```python
from build123d import *

# Parameters (mm, degrees)
SKETCH_1_W                    = 28.5
SKETCH_1_H                    = 8.75
EXTRUDE_1_DEPTH               = 1
HOLE_WIZARD_M10_1_D           = 11
HOLE_WIZARD_M10_1_CBORE_D     = 28.5
HOLE_WIZARD_M10_1_CBORE_DEPTH = 6.75
HOLE_WIZARD_2_5_2_5_1_D       = 2.5
HOLE_WIZARD_2_5_2_5_1_DEPTH   = 19.25
FILLET_1_R                    = 1


with BuildPart() as part:
    # 草图1 → 旋转1 (revolve)
    with BuildSketch(Plane.XZ, mode=Mode.PRIVATE) as revolve_1_sk:
        with Locations((14.25, 4.375)):
            Rectangle(SKETCH_1_W, SKETCH_1_H)
    revolve(revolve_1_sk.sketch.rotate(Axis((0, 0, 8.75), (0, 0, -1)), 180), axis=Axis((0, 0, 8.75), (0, 0, -1)))

    # 草图2 → 凸台-拉伸1 (add)
    with BuildSketch(Plane.XY.offset(8.75)):
        with BuildLine():
            Line((-8.705372964, 19.931858457), (-8.056820792, 17.511428803))
            ThreePointArc((-8.056820792, 17.511428803), (-5.758723754, 21.491849635), (-1.778302922, 19.193752596))
            Line((-1.778302922, 19.193752596), (-2.426855093, 21.614182251))
            ThreePointArc((-2.426855093, 21.614182251), (10.875, 18.836052532), (19.931858457, 8.705372964))
            Line((19.931858457, 8.705372964), (17.511428803, 8.056820792))
            ThreePointArc((17.511428803, 8.056820792), (21.491849635, 5.758723754), (19.193752596, 1.778302922))
            Line((19.193752596, 1.778302922), (21.614182251, 2.426855093))
            ThreePointArc((21.614182251, 2.426855093), (18.836052532, -10.875), (8.705372964, -19.931858457))
            Line((8.705372964, -19.931858457), (8.056820792, -17.511428803))
            ThreePointArc((8.056820792, -17.511428803), (5.758723754, -21.491849635), (1.778302922, -19.193752596))
            Line((1.778302922, -19.193752596), (2.426855093, -21.614182251))
            ThreePointArc((2.426855093, -21.614182251), (-10.875, -18.836052532), (-19.931858457, -8.705372964))
            Line((-19.931858457, -8.705372964), (-17.511428803, -8.056820792))
            ThreePointArc((-17.511428803, -8.056820792), (-21.491849635, -5.758723754), (-19.193752596, -1.778302922))
            Line((-19.193752596, -1.778302922), (-21.614182251, -2.426855093))
            ThreePointArc((-21.614182251, -2.426855093), (-18.836052532, 10.875), (-8.705372964, 19.931858457))
        make_face()
    extrude(amount=EXTRUDE_1_DEPTH)

    # 草图3 → 旋转2 (revolve)
    with BuildSketch(Plane.XZ, mode=Mode.PRIVATE) as revolve_2_sk:
        Polygon((8.5, 19.25), (0, 19.25), (0, 9.75), (9.5, 9.75), (9.5, 14.25), (8.5, 14.25), align=None)
    revolve(revolve_2_sk.sketch.rotate(Axis((0, 0, 19.25), (0, 0, -1)), 180), axis=Axis((0, 0, 19.25), (0, 0, -1)))

    # 草图4 → 切除-旋转1 (revolve, cut)
    with BuildSketch(Plane(origin=(0, -18.352590699, 0), x_dir=(1, 0, 0), z_dir=(0, 1, 0))):
        Polygon((6.617561857, 0), (4.917561857, 0), (4.917561857, -9.75), (8.167561857, -9.75), (8.167561857, -2.5), (6.617561857, -2.5), align=None)
    revolve(axis=Axis((4.917561857, -18.352590699, 0), (0, 0, 1)), mode=Mode.SUBTRACT)

    # 草图5 → 切除-旋转2 (revolve, cut)
    with BuildSketch(Plane(origin=(0, -4.917561857, 0), x_dir=(1, 0, 0), z_dir=(0, 1, 0))):
        Polygon((-16.652590699, 0), (-18.352590699, 0), (-18.352590699, -9.75), (-15.102590699, -9.75), (-15.102590699, -2.5), (-16.652590699, -2.5), align=None)
    revolve(axis=Axis((-18.352590699, -4.917561857, 0), (0, 0, 1)), mode=Mode.SUBTRACT)

    # 草图6 → 切除-旋转3 (revolve, cut)
    with BuildSketch(Plane(origin=(0, 18.352590699, 0), x_dir=(1, 0, 0), z_dir=(0, 1, 0))):
        Polygon((-3.217561857, 0), (-4.917561857, 0), (-4.917561857, -9.75), (-1.667561857, -9.75), (-1.667561857, -2.5), (-3.217561857, -2.5), align=None)
    revolve(axis=Axis((-4.917561857, 18.352590699, 0), (0, 0, 1)), mode=Mode.SUBTRACT)

    # 草图7 → 切除-旋转4 (revolve, cut)
    with BuildSketch(Plane(origin=(0, 4.917561857, 0), x_dir=(1, 0, 0), z_dir=(0, 1, 0))):
        Polygon((20.052590699, 0), (18.352590699, 0), (18.352590699, -9.75), (21.602590699, -9.75), (21.602590699, -2.5), (20.052590699, -2.5), align=None)
    revolve(axis=Axis((18.352590699, 4.917561857, 0), (0, 0, 1)), mode=Mode.SUBTRACT)

    # M10 六角头螺栓的柱形沉头孔1 (through all)
    with Locations(Plane(origin=(0, 0, 0), x_dir=(-1, 0, 0), z_dir=(0, 0, -1))):
        with Locations((0, 0)):
            CounterBoreHole(HOLE_WIZARD_M10_1_D / 2, HOLE_WIZARD_M10_1_CBORE_D / 2, HOLE_WIZARD_M10_1_CBORE_DEPTH)

    # Ø2.5 (2.5) 直径孔1
    with Locations(Plane(origin=(0, 0, 0), x_dir=(-1, 0, 0), z_dir=(0, 0, -1))):
        with Locations((-25, 0), (-12.5, 21.650635095), (12.5, 21.650635095), (25, 0), (12.5, -21.650635095), (-12.5, -21.650635095)):
            Hole(HOLE_WIZARD_2_5_2_5_1_D / 2, depth=HOLE_WIZARD_2_5_2_5_1_DEPTH)

    # 圆角1
    fillet_1_edges = [part.edges().sort_by_distance(p)[0] for p in [
        (-8.705372964, 19.931858457, 9.25),
        (-21.614182251, -2.426855093, 9.25),
        (-19.931858457, -8.705372964, 9.25),
        (2.426855093, -21.614182251, 9.25),
        (8.705372964, -19.931858457, 9.25),
        (21.614182251, 2.426855093, 9.25),
        (19.931858457, 8.705372964, 9.25),
        (-2.426855093, 21.614182251, 9.25),
    ]]
    fillet(fillet_1_edges, radius=FILLET_1_R)


solid = part.part
```
Part model, mm, in its own coordinate system. A direction names the side the tool comes from. Round coordinates to 2 decimals unless told otherwise and drop trailing zeros. Loops run counter-clockwise (first coordinate to the right, second up) from the corner with the lowest first, then second, coordinate; pieces in that order, holes last.
Item 1: Drop flat-ended pins along their axis: P1, Ø4, axis at y = 6, z = 5.5, coming from the +X side; P2, Ø5.5, axis at x = 4.92, y = -18.35, coming from the +Z side; P3, Ø5, axis at y = 13, z = 9, coming from the +X side. Give the stop position or say it passes through.
Item 2: Cut at B-B, the plane z = 8. State how many separate pieces and enclosed holes the cut face has, then the cut area to 3 significant figures.
Item 3: Drill centre lines: line 1 (Z direction, x = -1.5, y = 17); line 2 (Z direction, x = -11.5, y = -4); line 3 (Y direction, x = 12.5, z = 6.5). Where is each one in solid material? Low to high.
Item 4: 3-axis set-ups, long thin cutter, end or side, ignore diameter. For faces 1 (the face through (20, 4, 2.5)), 2 (the face through (19.923, 4.266, 1.232)): which of +Z, -Z, +X, -X, +Y, -Y reach the whole face in a straight line?
Item 5: Mould opens along X. For faces 3 (the face through (-7, 13, 0)), 4 (the face through (-13.163, -5.458, 3.328)), 5 (the face through (1.107, 8.428, 16.785)), 6 (the face through (18.924, -10.722, 9.243)) say: +X half, -X half, draft (parallel to the pull), parting line (faces both ways), or undercut.
Item 6: Cut at A-A, the plane x = 12.5. Give the cut face in (y, z).
Item 7: Cut at D-D, the plane x = 25. Give the cut face in (y, z).
Item 8: Cut at C-C, the plane z = 15.25. Give the cut face in (x, y), then the cut area to 3 significant figures.
A:
1. P1: stops at x = 28.22
1. P2: stops at z = 2.5
1. P3: stops at x = 26.49
2. separate pieces: 1
2. enclosed holes: 11
2. area: 2,290 mm2
3. line 1: z = 0 to 9.75
3. line 2: z = 6.75 to 9.75
3. line 3: y = -25.61 to -22.9, -20.4 to -6.84, 6.84 to 20.4, 22.9 to 25.61
4. face 1: +Z
4. face 2: +Z, -Z
5. face 3: draft
5. face 4: undercut
5. face 5: parting line
5. face 6: +X half
6. outline: (-25.61, 0) - (-22.9, 0) - (-22.9, 8.75) - (-25.61, 8.75) - close; (-20.4, 0) - (-6.84, 0) - (-6.84, 6.75) - (6.84, 6.75) - (6.84, 0) - (20.4, 0) - (20.4, 8.75) - (17.8, 8.75) - (17.8, 9.75) - (-17.8, 9.75) - (-17.8, 8.75) - (-20.4, 8.75) - close; (22.9, 0) - (25.61, 0) - (25.61, 8.75) - (22.9, 8.75) - close
7. outline: (-13.68, 0) - (-1.25, 0) - (-1.25, 8.75) - (-13.68, 8.75) - close; (1.25, 0) - (13.68, 0) - (13.68, 8.75) - (1.25, 8.75) - close
8. outline: circle Ø17 at (0, 0); hole circle Ø11 at (0, 0)
8. area: 132 mm2
